from build123d import *

# Parameters (mm, degrees)
BOSS_EXTRUDE3_DEPTH            = 1
SKETCH7_R                      = 10
BOSS_EXTRUDE4_DEPTH            = 0.75
SKETCH8_R                      = 3.5
BOSS_EXTRUDE5_DEPTH            = 1
SKETCH9_R                      = 1.75
BOSS_EXTRUDE6_DEPTH            = 1.1
SKETCH10_R                     = 1
BOSS_EXTRUDE7_DEPTH            = 6
F_1_6_1_6_DIAMETER_HOLE1_D     = 1.6
F_1_6_1_6_DIAMETER_HOLE1_DEPTH = 4.5
F_1_6_1_6_DIAMETER_HOLE1_TIP   = 0.480688495
SKETCH13_R                     = 9
BOSS_EXTRUDE8_DEPTH            = 2.3


with BuildPart() as part:
    # Sketch1 → Revolve1 (revolve)
    with BuildSketch(Plane(origin=(0, 0, 0), x_dir=(1, 0, 0), z_dir=(0, 1, 0))):
        Polygon((11, 0), (0, 0), (0, -23.45), (11, -23.45), (11, -2.020710678), (10.95, -2), (11, -1.979289322), (11, -0.620710678), (10.95, -0.6), (11, -0.579289322), align=None)
    revolve(axis=Axis((0, 0, 0), (0, 0, 1)))

    # Sketch6 → Boss-Extrude3 (add)
    with BuildSketch(Plane(origin=(0, 0, 0), x_dir=(-1, 0, 0), z_dir=(0, 0, -1))):
        with BuildLine():
            Line((5.05, 5.477225575), (5.05, -5.477225575))
            ThreePointArc((5.05, -5.477225575), (0, -7.45), (-5.05, -5.477225575))
            Line((-5.05, -5.477225575), (-5.05, 5.477225575))
            ThreePointArc((-5.05, 5.477225575), (0, 7.45), (5.05, 5.477225575))
        make_face()
    extrude(amount=BOSS_EXTRUDE3_DEPTH)

    # Sketch7 → Boss-Extrude4 (add)
    with BuildSketch(Plane.XY.offset(23.45)):
        Circle(SKETCH7_R)
    extrude(amount=BOSS_EXTRUDE4_DEPTH)

    # Sketch8 → Boss-Extrude5 (add)
    with BuildSketch(Plane.XY.offset(24.2)):
        Circle(SKETCH8_R)
    extrude(amount=BOSS_EXTRUDE5_DEPTH)

    # Sketch9 → Boss-Extrude6 (add)
    with BuildSketch(Plane.XY.offset(25.2)):
        Circle(SKETCH9_R)
    extrude(amount=BOSS_EXTRUDE6_DEPTH)

    # Sketch10 → Boss-Extrude7 (add)
    with BuildSketch(Plane.XY.offset(26.3)):
        Circle(SKETCH10_R)
    extrude(amount=BOSS_EXTRUDE7_DEPTH)

    # Ø1.6 (1.6) Diameter Hole1
    with Locations(Plane.XY.offset(24.2)):
        with Locations((-3, 5.196152423), (3, 5.196152423), (6, 0), (3, -5.196152423), (-3, -5.196152423), (-6, 0)):
            Hole(F_1_6_1_6_DIAMETER_HOLE1_D / 2, depth=F_1_6_1_6_DIAMETER_HOLE1_DEPTH)
            with Locations((0, 0, -(F_1_6_1_6_DIAMETER_HOLE1_DEPTH + F_1_6_1_6_DIAMETER_HOLE1_TIP / 2))):  # 118° drill point
                Cone(0, F_1_6_1_6_DIAMETER_HOLE1_D / 2, F_1_6_1_6_DIAMETER_HOLE1_TIP, mode=Mode.SUBTRACT)

    # Sketch13 → Boss-Extrude8 (add)
    with BuildSketch(Plane(origin=(0, 0, 0), x_dir=(-1, 0, 0), z_dir=(0, 0, -1))):
        Circle(SKETCH13_R)
    extrude(amount=BOSS_EXTRUDE8_DEPTH)


solid = part.part
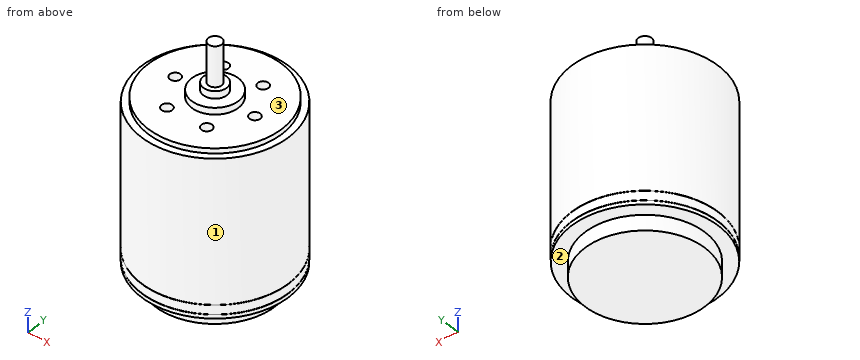
Input: part model. Units: mm. Frame: model coordinates. Face numbers are marked on the shaded views. A direction names the side the tool comes from. Give positions to 0.01 mm unless a question says otherwise; leave off trailing zeros. Order: outer loops, then holes, each group sorted by start corner. A loop starts at its lowest first (then second) coordinate and runs counter-clockwise, first axis right, second up. Notation, with made-up numbers: (83, -10.75) - (120, -10.75) arc R28 cw to (120, 19.25) - close; hole circle Ø7 at (80, 41). An arc over 180 degrees is marked (long way). Answer as a JSON object with one key per item and string values. Group by question number.
Q1. Cut plane B-B, the plane z = 5.5. Output: boundary loops of the cut face in (x, y), then the cut area to 3 significant figures.
Q2. First-contact query: pin 1 Ø2 at (x, y) = (3, -5.2) entering from +Z; pin 2 Ø1 at (x, z) = (5.5, 16.5) entering from -Y; pin 3 Ø12 at (y, z) = (7.5, 18) entering from +X. Flat tips, straight axial feed; report the tip coordinate or a pass-through.
Q3. Set-up query: the marked faces 1, 2 and 3. Return all of +Z, -Z, +X, -X, +Y, -Y with unobstructed straight access to the full face (end or side cutting, diameter ignored); none if empty.
Q4. Line query: probe 1 along Y at (x, z) = (3, 20.95); probe 2 along Z at (x, y) = (-3, -7); probe 3 along Z at (x, y) = (-8.25, -3.75). Output: solid intervals per line, ascending.
Q5. Cut plane A-A, the plane z = 29. Output: boundary loops of the cut face in (x, y).
Results:
{
 "1": {"outline": "circle Ø22 at (0, 0)", "area": "380 mm^2"},
 "2": {"pin 1": "z = 24.2", "pin 2": "y = -9.8", "pin 3": "x = 10.9"},
 "3": {"face 1": "+Z, -Z", "face 2": "-Z", "face 3": "+Z"},
 "4": {"probe 1": "-10.58 to -6, -4.4 to 4.4, 6 to 10.58", "probe 2": "-2.3 to 24.2", "probe 3": "0 to 24.2"},
 "5": {"outline": "circle Ø2 at (0, 0)"}
}
